Source: CAD feature listing. Evaluate the final solid. Frame: model axes, mm. Round coordinates to 2 decimals unless told otherwise and drop trailing zeros. Write each loop counter-clockwise with the first axis right and the second up, starting at its lowest first coordinate (ties: lowest second). Pieces come first, ordered by that corner, then holes.
```python
from build123d import *

# Parameters (mm, degrees)
BOSS_EXTRUDE1_DEPTH = 4.7625


with BuildPart() as part:
    # Sketch1 → Boss-Extrude1 (new body)
    with BuildSketch(Plane.XY):
        Polygon((-22.0345, -16.51), (-1.7, -16.51), (-1.7, -14.01), (-2.75, -14.01), (-2.75, -11.01), (-1.7, -11.01), (-1.7, -8.51), (1.7, -8.51), (1.7, -11.01), (2.75, -11.01), (2.75, -14.01), (1.7, -14.01), (1.7, -16.51), (22.0345, -16.51), (22.0345, 16.51), (1.7, 16.51), (1.7, 14.01), (2.75, 14.01), (2.75, 11.01), (1.7, 11.01), (1.7, 8.51), (-1.7, 8.51), (-1.7, 11.01), (-2.75, 11.01), (-2.75, 14.01), (-1.7, 14.01), (-1.7, 16.51), (-22.0345, 16.51), align=None)
    extrude(amount=BOSS_EXTRUDE1_DEPTH)


solid = part.part
```
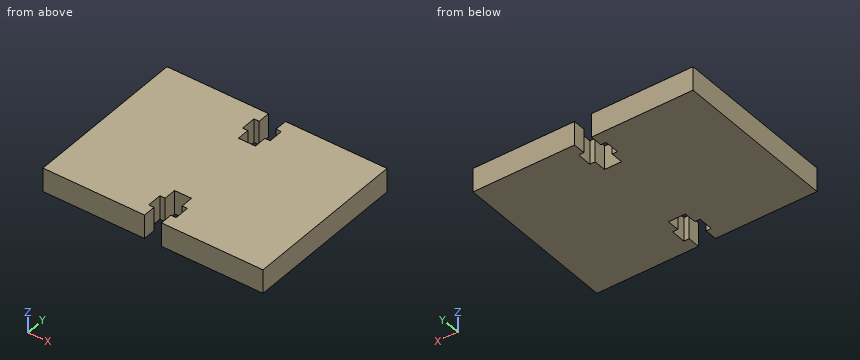
Q1. Pin query (flat end, axial travel): P1, Ø1.7, axis at x = 0, z = 2.5, coming from the +Y side. Return the tip coordinate at first contact, or that it passes through.
Q2. Section query A-A, the plane y = -10. Output: boundary loops of the cut face in (x, z), and give its area (3 significant figures).
Q3. Line query: line 1 (X direction, y = 10.5, z = 1.1); line 2 (Y direction, x = 1, z = 1). Output: solid intervals per line, ascending.
Q4. Section query B-B, the plane z = 0.55. Output: boundary loops of the cut face in (x, y), and give its area (3 significant figures).
Filled in:
1. P1: stops at y = 8.51
2. outline: (-22.03, 0) - (-1.7, 0) - (-1.7, 4.76) - (-22.03, 4.76) - close; (1.7, 0) - (22.03, 0) - (22.03, 4.76) - (1.7, 4.76) - close
2. area: 194 mm2
3. line 1: x = -22.03 to -1.7, 1.7 to 22.03
3. line 2: y = -8.51 to 8.51
4. outline: (-22.03, -16.51) - (-1.7, -16.51) - (-1.7, -14.01) - (-2.75, -14.01) - (-2.75, -11.01) - (-1.7, -11.01) - (-1.7, -8.51) - (1.7, -8.51) - (1.7, -11.01) - (2.75, -11.01) - (2.75, -14.01) - (1.7, -14.01) - (1.7, -16.51) - (22.03, -16.51) - (22.03, 16.51) - (1.7, 16.51) - (1.7, 14.01) - (2.75, 14.01) - (2.75, 11.01) - (1.7, 11.01) - (1.7, 8.51) - (-1.7, 8.51) - (-1.7, 11.01) - (-2.75, 11.01) - (-2.75, 14.01) - (-1.7, 14.01) - (-1.7, 16.51) - (-22.03, 16.51) - close
4. area: 1,390 mm2
